```python
from build123d import *

# Parameters (mm, degrees)
FILLET1_R     = 0.396875
CHAMFER1_SIZE = 0.254


with BuildPart() as part:
    # Sketch1 → Revolve1 (revolve)
    with BuildSketch(Plane.XY):
        Polygon((1.5875, 0), (6.0325, 0), (6.0325, 3.175), (2.921, 3.175), (2.921, 12.7), (1.5875, 12.7), align=None)
    revolve(axis=Axis((0, 7.886499903, 0), (0, -1, 0)))

    # Fillet1
    fillet1_edges = [part.edges().sort_by_distance(p)[0] for p in [
        (-2.921, 3.175, 0),
    ]]
    fillet(fillet1_edges, radius=FILLET1_R)

    # Chamfer1
    chamfer1_edges = [part.edges().sort_by_distance(p)[0] for p in [
        (-1.5875, 12.7, 0),
        (-2.921, 12.7, 0),
        (-6.0325, 3.175, 0),
        (-6.0325, 0, 0),
        (-1.5875, 0, 0),
    ]]
    chamfer(chamfer1_edges, length=CHAMFER1_SIZE)


solid = part.part
```
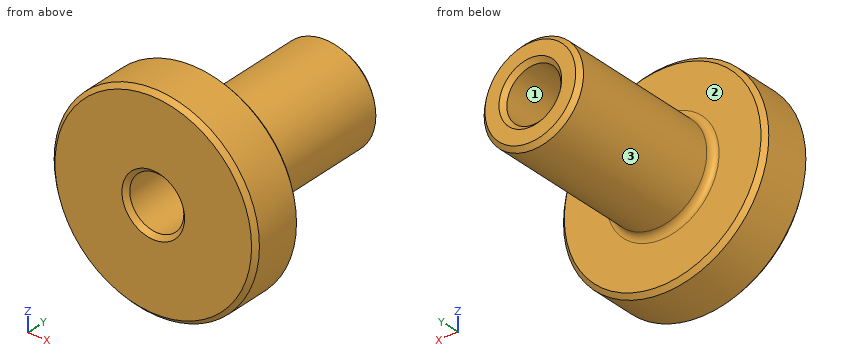
Check sheet for the modelled part. Datum: model origin and axes. Units: mm. Face numbers are marked on the shaded views. Give positions to 0.01 mm unless a question says otherwise; leave off trailing zeros. Write each loop counter-clockwise with the first axis right and the second up, starting at its lowest first coordinate (ties: lowest second). Pieces come first, ordered by that corner, then holes.
Item 1: Draft check along X on the marked faces 1, 2 and 3. Enter one of: released by +X, released by -X, zero draft, split by the parting line, or undercut.
Item 2: Scan lines: L1, parallel to Z at x = 0, y = 7.5; L2, parallel to Z at x = 0, y = 2.75; L3, parallel to Y at x = 1, z = 5.5 (3 decimals). Record each from-to range of solid material in increasing order.
Item 3: Cross-section at C-C (y = 2). Enter the section's corners in (x, z) (1 decimal).
Item 4: Cross-section at D-D (y = 4.25). Enter the section's corners in (x, z) (1 decimal).
Item 5: Gauge pin test, flat ends, axial feed: pin 1 (5 mm diameter, centred on y = 10.5, z = -4.5, fed in from +X); pin 2 (1.5 mm diameter, centred on y = 9.5, z = -2.5, fed in from +X); pin 3 (3 mm diameter, centred on y = 6.5, z = 1.5, fed in from -X); pin 4 (1.9 mm diameter, centred on x = 0, z = 0, fed in from +Y). Record the tip position at first contact, or that the pin passes through.
Report:
1. face 1: undercut
1. face 2: zero draft
1. face 3: split by the parting line
2. L1: z = -2.92 to -1.59, 1.59 to 2.92
2. L2: z = -6.03 to -1.59, 1.59 to 6.03
2. L3: y = 0 to 3.175
3. outline: circle Ø12.1 at (0, 0); hole circle Ø3.2 at (0, 0)
4. outline: circle Ø5.8 at (0, 0); hole circle Ø3.2 at (0, 0)
5. pin 1: stops at x = 2.13
5. pin 2: stops at x = 2.34
5. pin 3: stops at x = -2.92
5. pin 4: passes through
